Read the model definition and answer for the solid it produces. Units are mm, in the model's axes. Give positions to 0.01 mm unless a question says otherwise; leave off trailing zeros. Loops run counter-clockwise (first coordinate to the right, second up) from the corner with the lowest first, then second, coordinate; pieces in that order, holes last. Notation, with made-up numbers: (4.5, 17.5) - (23.5, 17.5) arc R35 ccw to (23.5, 49.5) - close; hole circle Ø7 at (87, -21). An arc over 180 degrees is marked (long way). Use a Markdown table: item, result. Add a question column.
Item 1: A cutting plane is placed at A-A (z = 0). Determine the outline of the cut face in (x, y), plus the area to 3 significant figures.
Item 2: A cutting plane is placed at B-B (x = 0). Determine the outline of the cut face in (y, z), plus the area to 3 significant figures.
Item 3: Consider probe 1 along X at (y, z) = (7.25, 0); probe 2 along X at (y, z) = (5.75, 59.5). Determine where each line is inside the solid, lowest interval first. Write a range as [from, to].
Item 4: Each of these flat-tipped pins is pushed along its axis until it touches: P1, Ø6, axis at y = 10, z = 46.5, coming from the -X side; P2, Ø2, axis at y = 9.5, z = 62.5, coming from the +X side; P3, Ø1.5, axis at y = 9, z = 46, coming from the +X side. Where does it stop, or does it pass through?
Item 5: A cutting plane is placed at C-C (y = 6.75). Give the number of separate pieces and of enclosed holes in the cut face, plus the area to 3 significant figures.
from build123d import *

# Parameters (mm, degrees)
SKETCH2_W                = 82.55
SKETCH2_H                = 12.7
CUT_EXTRUDE1_DEPTH       = 13.7
FILLET1_R                = 4
CIRPATTERN4_COUNT        = 8
FILLET1_OF_CIRPATTERN4_R = 4
SKETCH9_R                = 33
CUT_EXTRUDE2_DEPTH       = 13.7
SKETCH10_R               = 84.55
SKETCH10_R_2             = 82.55
BOSS_EXTRUDE1_DEPTH      = 12.7


with BuildPart() as part:
    # Sketch2 → Revolve1 (revolve)
    with BuildSketch(Plane(origin=(0, 0, 0), x_dir=(0, 0, -1), z_dir=(1, 0, 0))):
        with Locations((-41.275, 6.35)):
            Rectangle(SKETCH2_W, SKETCH2_H)
    revolve(axis=Axis((0, -0.5, 0), (0, 1, 0)))

    # Sketch8 → Cut-Extrude1 (cut, through all)
    with BuildSketch(Plane(origin=(0, 12.7, 0), x_dir=(1, 0, 0), z_dir=(0, 1, 0))):
        with BuildLine():
            Line((-10.567880231, 38.578749428), (-24.995954941, 73.411203073))
            ThreePointArc((-24.995954941, 73.411203073), (0, 77.55), (24.995954941, 73.411203073))
            Line((24.995954941, 73.411203073), (10.567880231, 38.578749428))
            ThreePointArc((10.567880231, 38.578749428), (0, 40), (-10.567880231, 38.578749428))
        make_face()
    cut_extrude1 = extrude(amount=-CUT_EXTRUDE1_DEPTH, mode=Mode.SUBTRACT)

    # Fillet1
    fillet1_edges = [part.edges().sort_by_distance(p)[0] for p in [
        (10.567880231, 6.35, -38.578749428),
        (-10.567880231, 6.35, -38.578749428),
        (-24.995954941, 6.35, -73.411203073),
        (24.995954941, 6.35, -73.411203073),
    ]]
    fillet(fillet1_edges, radius=FILLET1_R)

    # CirPattern4: Cut-Extrude1 ×8 about axis
    cirpattern4_axis = Axis((0, 0, 0), (0, 1, 0))
    for i in range(1, CIRPATTERN4_COUNT):
        add(cut_extrude1.rotate(cirpattern4_axis, i * 360 / CIRPATTERN4_COUNT), mode=Mode.SUBTRACT)

    # Fillet1 of CirPattern4
    fillet1_of_cirpattern4_edges = [part.edges().sort_by_distance(p)[0] for p in [
        (-19.806675556, 6.35, -34.751915104),
        (-34.751915104, 6.35, -19.806675556),
        (-69.584368749, 6.35, -34.234750266),
        (-34.234750266, 6.35, -69.584368749),
        (-38.578749428, 6.35, -10.567880231),
        (-38.578749428, 6.35, 10.567880231),
        (-73.411203073, 6.35, 24.995954941),
        (-73.411203073, 6.35, -24.995954941),
        (-34.751915104, 6.35, 19.806675556),
        (-19.806675556, 6.35, 34.751915104),
        (-34.234750266, 6.35, 69.584368749),
        (-69.584368749, 6.35, 34.234750266),
        (-10.567880231, 6.35, 38.578749428),
        (10.567880231, 6.35, 38.578749428),
        (24.995954941, 6.35, 73.411203073),
        (-24.995954941, 6.35, 73.411203073),
        (19.806675556, 6.35, 34.751915104),
        (34.751915104, 6.35, 19.806675556),
        (69.584368749, 6.35, 34.234750266),
        (34.234750266, 6.35, 69.584368749),
        (38.578749428, 6.35, 10.567880231),
        (38.578749428, 6.35, -10.567880231),
        (73.411203073, 6.35, -24.995954941),
        (73.411203073, 6.35, 24.995954941),
        (34.751915104, 6.35, -19.806675556),
        (19.806675556, 6.35, -34.751915104),
        (34.234750266, 6.35, -69.584368749),
        (69.584368749, 6.35, -34.234750266),
    ]]
    fillet(fillet1_of_cirpattern4_edges, radius=FILLET1_OF_CIRPATTERN4_R)

    # Sketch9 → Cut-Extrude2 (cut, through all)
    with BuildSketch(Plane(origin=(0, 12.7, 0), x_dir=(1, 0, 0), z_dir=(0, 1, 0))):
        Circle(SKETCH9_R)
    extrude(amount=-CUT_EXTRUDE2_DEPTH, mode=Mode.SUBTRACT)

    # Sketch10 → Boss-Extrude1 (add)
    with BuildSketch(Plane(origin=(0, 0, 0), x_dir=(1, 0, 0), z_dir=(0, 1, 0))):
        Circle(SKETCH10_R)
        Circle(SKETCH10_R_2, mode=Mode.SUBTRACT)
    extrude(amount=BOSS_EXTRUDE1_DEPTH)


solid = part.part
Geometry says:
| question | item | result |
|---|---|---|
| 1 | outline | (-84.55, 0) - (-77.55, 0) - (-77.55, 12.7) - (-84.55, 12.7) - close; (-40, 0) - (-33, 0) - (-33, 12.7) - (-40, 12.7) - close; (33, 0) - (40, 0) - (40, 12.7) - (33, 12.7) - close; (77.55, 0) - (84.55, 0) - (84.55, 12.7) - (77.55, 12.7) - close |
| 1 | area | 356 mm² |
| 2 | outline | (0, -84.55) - (12.7, -84.55) - (12.7, -77.55) - (0, -77.55) - close; (0, -40) - (12.7, -40) - (12.7, -33) - (0, -33) - close; (0, 33) - (12.7, 33) - (12.7, 40) - (0, 40) - close; (0, 77.55) - (12.7, 77.55) - (12.7, 84.55) - (0, 84.55) - close |
| 2 | area | 356 mm² |
| 3 | probe 1 | [-84.55, -77.55], [-40, -33], [33, 40], [77.55, 84.55] |
| 3 | probe 2 | [-60.07, -49.74], [-30.06, -19.23], [19.23, 30.06], [49.74, 60.07] |
| 4 | P1 | x = -72.5 |
| 4 | P2 | x = 58.02 |
| 4 | P3 | x = 71.42 |
| 5 | separate pieces | 1 |
| 5 | enclosed holes | 9 |
| 5 | area | 8,280 mm² |
